Here's how the part is built. I have some questions about the finished solid (model axes, mm). Face numbers are marked on the shaded views. A direction names the side the tool comes from. Give positions to 0.01 mm unless a question says otherwise; leave off trailing zeros. Write each loop counter-clockwise with the first axis right and the second up, starting at its lowest first coordinate (ties: lowest second). Pieces come first, ordered by that corner, then holes. Notation, with made-up numbers: (11, 67) -> (33, 67) arc R31 ccw to (33, 105) -> close; hole circle Ø2 at (-0.75, 10.5). An arc over 180 degrees is marked (long way). Return JSON: item names as keys, results as strings.
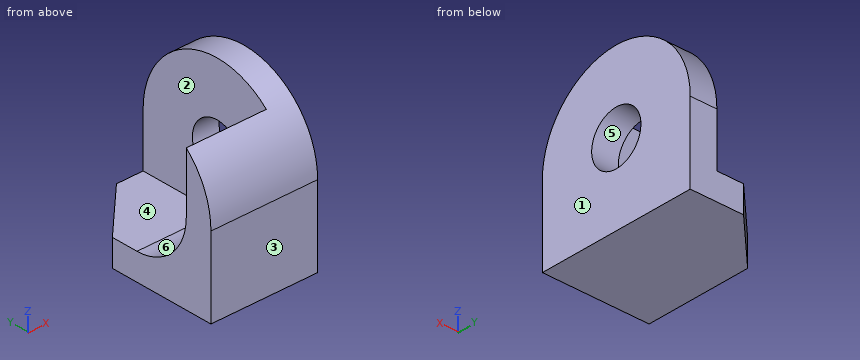
from build123d import *

# Parameters (mm, degrees)
BOSS_EXTRUDE1_DEPTH      = 1
BOSS_EXTRUDE1_DEPTH_BACK = 3
SKETCH1_R                = 1
CUT_EXTRUDE2_DEPTH       = 3
CHAMFER1_SIZE            = 2


with BuildPart() as part:
    # Sketch1 → Boss-Extrude1 (new, two sides: drawn at the far end of the back side and taken through both)
    with BuildSketch(Plane(origin=(0, 0, 0), x_dir=(0, 0, -1), z_dir=(1, 0, 0)).offset(-BOSS_EXTRUDE1_DEPTH_BACK)):
        with BuildLine():
            Line((0, 0), (0, 6))
            Line((0, 6), (-3, 6))
            ThreePointArc((-3, 6), (-6, 3), (-3, 0))
            Line((-3, 0), (0, 0))
        make_face()
        with Locations((-3, 3)):
            Circle(SKETCH1_R, mode=Mode.SUBTRACT)
    extrude(amount=BOSS_EXTRUDE1_DEPTH + BOSS_EXTRUDE1_DEPTH_BACK)

    # Sketch2 → Cut-Extrude2 (cut)
    with BuildSketch(Plane.ZY.offset(3)):
        with BuildLine():
            Line((3, 1), (7.614070683, 1))
            Line((7.614070683, 1), (7.614070683, 6.174190234))
            Line((7.614070683, 6.174190234), (1, 6.174190234))
            Line((1, 6.174190234), (1, 4.020419478))
            Line((1, 4.020419478), (1, 3))
            ThreePointArc((1, 3), (1.585786438, 1.585786438), (3, 1))
        make_face()
    extrude(amount=-CUT_EXTRUDE2_DEPTH, mode=Mode.SUBTRACT)

    # Chamfer1
    chamfer1_edges = [part.edges().sort_by_distance(p)[0] for p in [
        (-3, 6, 0.5),
    ]]
    chamfer(chamfer1_edges, length=CHAMFER1_SIZE)


solid = part.part
1. For pin 1 Ø0.9 at (x, y) = (-2, 4) entering from +Z; pin 2 Ø2.5 at (y, z) = (3, 3) entering from -X; pin 3 Ø1.1 at (x, z) = (-1.5, 3.5) entering from +Y, each with a flat end and sliding along its axis, tell me the tip position at first contact or that it passes through.
Taken from the geometry:
{"pin 1": "stops at z = 1", "pin 2": "stops at x = 0", "pin 3": "stops at y = 1"}
2. If I drill on line 1 (Z direction, x = 0.6, y = 3); line 2 (X direction, y = 5, z = 3.3), over which ranges is the centre line in solid material (lowest first)? Write a range as [from, to].
Taken from the geometry:
{"line 1": "z = [0, 2], [4, 6]", "line 2": "x = [0, 1]"}
3. Which directions (+Z, -Z, +X, -X, +Y, -Y) give clear straight access to the entire face, cutting with the end or side of a thin tool? Please do the marked faces 1 and 2.
Taken from the geometry:
{"face 1": "+Z, -Z, +X, +Y, -Y", "face 2": "+Z, -X, +Y"}
4. If we mould it in two halves opening along Y, with no side actions, what happens to the marked faces 3, 4, 5 and 6? For each: released by +Y, released by -Y, zero draft, split by the parting line, or undercut.
Taken from the geometry:
{"face 3": "released by -Y", "face 4": "zero draft", "face 5": "undercut", "face 6": "released by +Y"}
5. Suppose I cut it at D-D, the plane y = 4.45. List the corners of the cut face in (x, z) for me, and give its area (3 significant figures).
Taken from the geometry:
{"outline": "(-2.55, 0) -> (1, 0) -> (1, 5.63) -> (0, 5.63) -> (0, 1) -> (-2.55, 1) -> close", "area": "8.18 mm²"}
6. Suppose I cut it at B-B, the plane x = -1.15. List the corners of the cut face in (y, z) for me.
Taken from the geometry:
{"outline": "(0, 0) -> (5.85, 0) -> (5.85, 1) -> (3, 1) arc R2 cw to (1, 3) -> (1, 5.24) arc R3 ccw to (0, 3) -> close"}
7. Suppose I cut it at A-A, the plane y = 3.8. List the corners of the cut face in (x, z) for me.
Taken from the geometry:
{"outline": "(-3, 0) -> (1, 0) -> (1, 2.4) -> (0, 2.4) -> (0, 1) -> (-3, 1) -> close; (0, 3.6) -> (1, 3.6) -> (1, 5.89) -> (0, 5.89) -> close"}
8. Suppose I cut it at C-C, the plane z = 0.9. List the corners of the cut face in (x, y) for me, and give its area (3 significant figures).
Taken from the geometry:
{"outline": "(-3, 0) -> (1, 0) -> (1, 6) -> (-1, 6) -> (-3, 4) -> close", "area": "22.0 mm²"}
